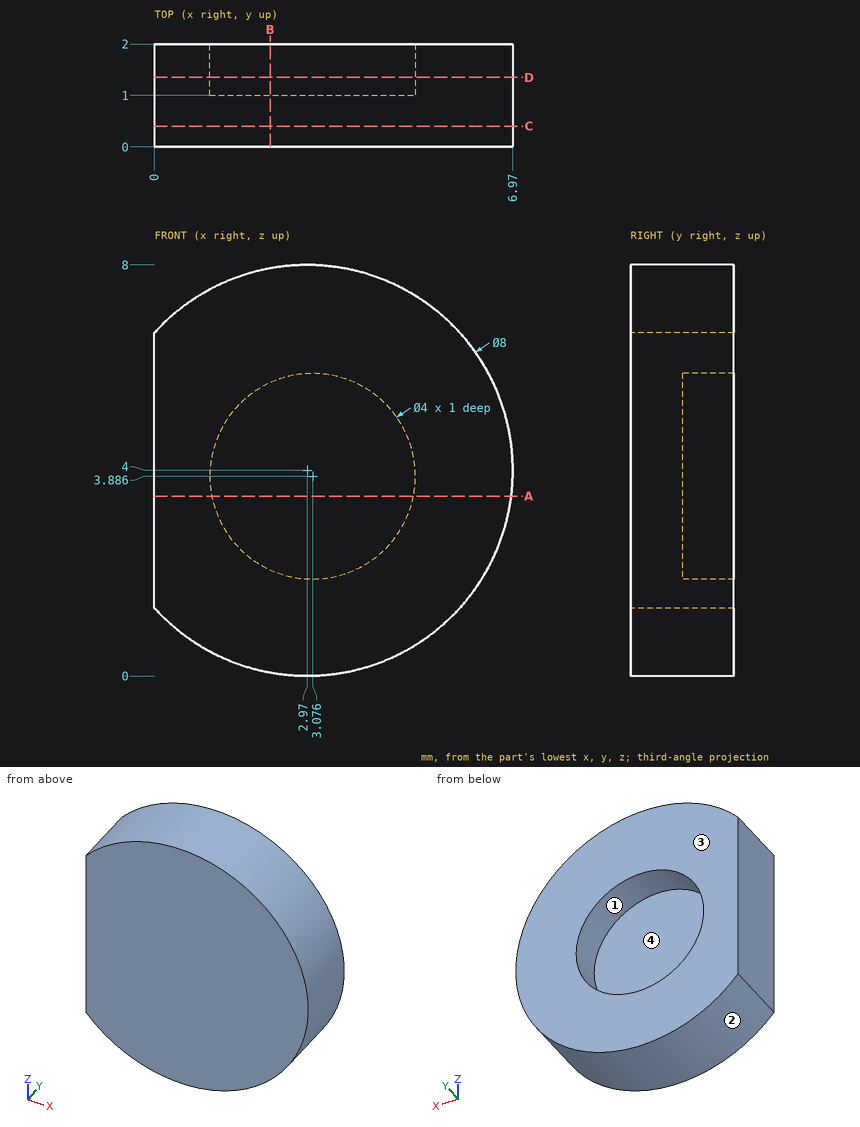
Source: three-view drawing plus pictorial views. Frame: mm from the lowest corner of the part. Give positions to 0.01 mm unless a question says otherwise; leave off trailing zeros. Loops run counter-clockwise (first coordinate to the right, second up) from the corner with the lowest first, then second, coordinate; pieces in that order, holes last. Notation, with made-up numbers: (23, 56.25) -> (81, 56.25) arc R29 ccw to (81, 90.25) -> close; hole circle Ø3 at (4.5, 59.5). An arc over 180 degrees is marked (long way). Put each result on its own line as item: value. Start each with the question number.
1) Material intervals for probe 1 along X at (y, z) = (0.25, 2.5); probe 2 along Y at (x, z) = (2, 2.25); probe 3 along Z at (x, y) = (3, 1.2) (1 decimal), sorted ascending.
2) Contact query for flat-ended pins moving along their axis: P1, Ø1, axis at y = 1.5, z = 5, coming from the +X side; P2, Ø1.2, axis at x = 2.5, z = 5, coming from the +Y side. Output: stop coordinate, or through.
3) Cut plane C-C (y = 0.4). Return loops of the section in (x, z), then the cut area to 3 significant figures.
4) Cut plane D-D (y = 1.35). Return loops of the section in (x, z).
5) Draft query along Z for the marked faces 1, 2, 3 and 4. Return one class per face: released by +Z, released by -Z, zero draft, split by the parting line, or undercut.
6) Cut plane A-A (z = 3.5). Return loops of the section in (x, y).
7) Cut plane B-B (x = 2.25). Return loops of the section in (y, z) (1 decimal).
Results are:
1. probe 1: x = 0 to 6.68
1. probe 2: y = 0 to 1
1. probe 3: z = 0 to 1.9, 5.9 to 8
2. P1: stops at x = 6.94
2. P2: stops at y = 1
3. outline: (0, 1.32) arc R4 ccw (long way) to (0, 6.68) -> close
3. area: 46.5 mm2
4. outline: (0, 1.32) arc R4 ccw (long way) to (0, 6.68) -> close; hole circle Ø4 at (3.08, 3.89)
5. face 1: undercut
5. face 2: split by the parting line
5. face 3: zero draft
5. face 4: undercut
6. outline: (0, 0) -> (6.94, 0) -> (6.94, 2) -> (5.04, 2) -> (5.04, 1) -> (1.11, 1) -> (1.11, 2) -> (0, 2) -> close
7. outline: (0, 0.1) -> (2, 0.1) -> (2, 2.1) -> (1, 2.1) -> (1, 5.7) -> (2, 5.7) -> (2, 7.9) -> (0, 7.9) -> close
